Design review of the part built by this model. Coordinates are the model's own, in mm. A direction names the side the tool comes from. Coordinates: 2 decimals unless noted, no trailing zeros. Write each loop counter-clockwise with the first axis right and the second up, starting at its lowest first coordinate (ties: lowest second). Pieces come first, ordered by that corner, then holes.
Q1. Take a section at A-A, the plane z = 0.45. Write out the cut boundary in (x, y) (1 decimal).
Q2. Take a section at B-B, the plane x = -6.5. Write out the cut boundary in (y, z).
Q3. For faces 5 (the flat face through (-4.71, -4.29, 0.3)), 6 (the flat face through (0, 0, 0.6)), 7 (the flat face through (4.29, -4.72, 0.3)), 8 (the flat face through (4.83, -4.41, 0.3)), 9 (the flat face through (4.409, 4.832, 0.296)), list the 3-axis set-ups (+Z, -Z, +X, -X, +Y, -Y) from which the entire face can be reached by the end or side of a thin tool; tool diameter is ignored.
Q4. Take a section at C-C, the plane y = 6.75. Write out the cut boundary in (x, z).
Q5. For L1, parallel to Y at x = -0.75, z = 0.5; L2, parallel to Y at x = 6, z = 0.1; L3, parallel to X at y = -7.5, z = 0.1, list the stretches that pass through material, from the lowest coordinate up.
Q6. The part is to be moulded in two halves that separate along Y. For faces 1 (the flat face through (-4.41, -4.84, 0.3)), 2 (the flat face through (-4.833, 4.407, 0.296)), 3 (the flat face through (4.711, 4.286, 0.296)), 4 (the flat face through (0, 0, 0)), say which applies: released by +Y, released by -Y, zero draft, split by the parting line, or undercut.
from build123d import *

# Parameters (mm, degrees)
F1_DEPTH = 0.6


with BuildPart() as f1:
    # F0 (on Top) → F1 (new body)
    with BuildSketch(Plane.XY):
        Polygon((-9.12, 9.12), (-9.12, 8.6956777771), (-0.4242059384, -0.0025), (-0.2121029692, 0.2096611115), align=None)
        Polygon((0.2121029692, -0.2146611115), (9.12, -9.125), (9.12, -8.7006777771), (0.4242059384, -0.0025), align=None)
        Polygon((-0.2121029692, 0.2096611115), (0, -0.0025), (0.2121029692, 0.2096611115), (0, 0.4218222229), align=None)
        Polygon((0, -0.4268222229), (8.6957940616, -9.125), (9.12, -9.125), (0.2121029692, -0.2146611115), align=None)
        Polygon((-8.6957940616, 9.12), (-9.12, 9.12), (-0.2121029692, 0.2096611115), (0, 0.4218222229), align=None)
        Polygon((0, -0.0025), (-0.2121029692, -0.2146611115), (0, -0.4268222229), (0.2121029692, -0.2146611115), align=None)
        Polygon((-0.4242059384, -0.0025), (-0.2121029692, -0.2146611115), (0, -0.0025), (-0.2121029692, 0.2096611115), align=None)
        Polygon((-0.2121029692, -0.2146611115), (-9.12, -9.125), (-8.6957940616, -9.125), (0, -0.4268222229), align=None)
        Polygon((9.12, 9.12), (0.2121029692, 0.2096611115), (0.4242059384, -0.0025), (9.12, 8.6956777771), align=None)
        Polygon((-9.12, -8.7006777771), (-9.12, -9.125), (-0.2121029692, -0.2146611115), (-0.4242059384, -0.0025), align=None)
        Polygon((0.2121029692, 0.2096611115), (0, -0.0025), (0.2121029692, -0.2146611115), (0.4242059384, -0.0025), align=None)
        Polygon((0, 0.4218222229), (0.2121029692, 0.2096611115), (9.12, 9.12), (8.6957940616, 9.12), align=None)
    extrude(amount=F1_DEPTH)


solid = f1.part
Responses:
1. outline: (-9.1, -9.1) - (-8.7, -9.1) - (0, -0.4) - (8.7, -9.1) - (9.1, -9.1) - (9.1, -8.7) - (0.4, 0) - (9.1, 8.7) - (9.1, 9.1) - (8.7, 9.1) - (0, 0.4) - (-8.7, 9.1) - (-9.1, 9.1) - (-9.1, 8.7) - (-0.4, 0) - (-9.1, -8.7) - close
2. outline: (-6.93, 0) - (-6.08, 0) - (-6.08, 0.6) - (-6.93, 0.6) - close; (6.07, 0) - (6.92, 0) - (6.92, 0.6) - (6.07, 0.6) - close
3. face 5: +Z, -Z, -X
3. face 6: +Z, +X, -X, +Y, -Y
3. face 7: +Z, -Z, -Y
3. face 8: +Z, -Z, +X
3. face 9: +Z, -Z, +Y
4. outline: (-7.17, 0) - (-6.33, 0) - (-6.33, 0.6) - (-7.17, 0.6) - close; (6.33, 0) - (7.17, 0) - (7.17, 0.6) - (6.33, 0.6) - close
5. L1: y = -1.18 to -0.33, 0.32 to 1.17
5. L2: y = -6.43 to -5.58, 5.57 to 6.42
5. L3: x = -7.92 to -7.07, 7.07 to 7.92
6. face 1: released by -Y
6. face 2: undercut
6. face 3: undercut
6. face 4: zero draft
